Check sheet for the modelled part. Datum: model origin and axes. Units: mm. Face numbers are marked on the shaded views. A direction names the side the tool comes from. Give positions to 0.01 mm unless a question says otherwise; leave off trailing zeros. Loops run counter-clockwise (first coordinate to the right, second up) from the corner with the lowest first, then second, coordinate; pieces in that order, holes last. Notation, with made-up numbers: (55.5, 18) -> (69.5, 18) arc R37 cw to (69.5, 54) -> close; hole circle Ø6 at (23.25, 38.25). An arc over 180 degrees is marked (long way). Write each question's results on one line, items separated by ' | '. Start each with the question number.
Item 1: Cross-section at C-C on z = 18. Enter the section's corners in (x, y), then the cut area to 3 significant figures.
Item 2: Access from +Z, -Z, +X, -X, +Y, -Y to the whole of each face (thin tool, end or side, straight path). Record for the marked faces 1, 2 and 3.
Item 3: Mould release check, pull along Z, two halves, no side actions. Record for the marked faces 4, 5, 6 and 7: pulls with the +Z half, pulls with the -Z half, needs draft (parallel to the pull), parting line crosses it, or undercut.
Item 4: Cross-section at A-A on x = 57. Enter the section's corners in (y, z).
Item 5: Cross-section at D-D on x = -60. Enter the section's corners in (y, z).
Item 6: Gauge pin test, flat ends, axial feed: pin 1 Ø6 at (x, z) = (-60, 25) entering from +Y; pin 2 Ø1 at (x, z) = (51, 36) entering from +Y; pin 3 Ø1 at (y, z) = (37.5, 41.5) entering from +X; pin 4 Ø20 at (y, z) = (41.5, 14) entering from -X. Record the tip position at first contact, or that the pin passes through.
Item 7: Cross-section at B-B on z = 25. Enter the section's corners in (x, y), then the cut area to 3 significant figures.
Item 8: Scan lines: line 1 along Z through (x, y) = (-60, 1); line 2 along Y through (x, z) = (0, 24.5); line 3 along Y through (x, z) = (-20, 13). Record each from-to range of solid material in increasing order.
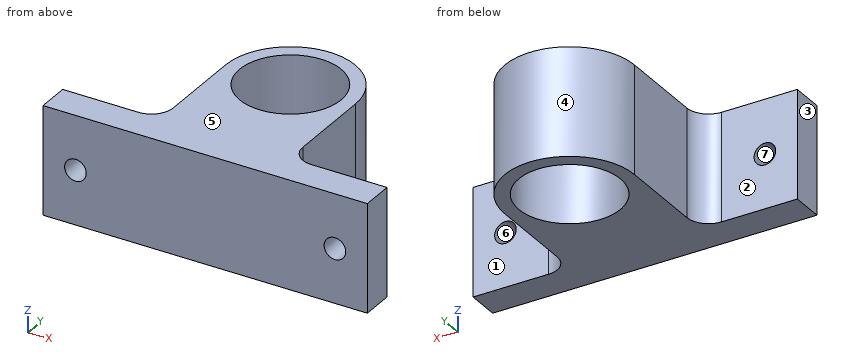
from build123d import *

# Parameters (mm, degrees)
IZIM1_R                     = 23.5
Y_KSEKLIK_EKSTR_ZYON1_DEPTH = 50
RADYUS1_R                   = 10
IZIM2_R                     = 5
KES_EKSTR_ZYON1_DEPTH       = 50


with BuildPart() as part:
    # Çizim1 → Yükseklik-Ekstrüzyon1 (new body)
    with BuildSketch(Plane.XY):
        with BuildLine():
            Line((-30, 7.5), (-30, 57.5))
            ThreePointArc((-30, 57.5), (0, 87.5), (30, 57.5))
            Line((30, 57.5), (30, 7.5))
            Line((30, 7.5), (75, 7.5))
            Line((75, 7.5), (75, -7.5))
            Line((75, -7.5), (-75, -7.5))
            Line((-75, -7.5), (-75, 7.5))
            Line((-75, 7.5), (-30, 7.5))
        make_face()
        with Locations((0, 57.5)):
            Circle(IZIM1_R, mode=Mode.SUBTRACT)
    extrude(amount=Y_KSEKLIK_EKSTR_ZYON1_DEPTH)

    # Radyus1
    radyus1_edges = [part.edges().sort_by_distance(p)[0] for p in [
        (-30, 7.5, 25),
        (30, 7.5, 25),
    ]]
    fillet(radyus1_edges, radius=RADYUS1_R)

    # Çizim2 → Kes-Ekstrüzyon1 (cut)
    with BuildSketch(Plane(origin=(0, 7.5, 0), x_dir=(1, 0, 0), z_dir=(0, 1, 0))):
        with Locations(Location((-60, -25, 0), (0, 0, 180))):
            Circle(IZIM2_R)
        with Locations(Location((60, -25, 0), (0, 0, 180))):
            Circle(IZIM2_R)
    extrude(amount=-KES_EKSTR_ZYON1_DEPTH, mode=Mode.SUBTRACT)


solid = part.part
Answer sheet:
1) outline: (-75, -7.5) -> (75, -7.5) -> (75, 7.5) -> (40, 7.5) arc R10 cw to (30, 17.5) -> (30, 57.5) arc R30 ccw to (-30, 57.5) -> (-30, 17.5) arc R10 cw to (-40, 7.5) -> (-75, 7.5) -> close; hole circle Ø47 at (0, 57.5) | area: 4,970 mm²
2) face 1: +Z, -Z, +X, +Y | face 2: +Z, -Z, -X, +Y | face 3: +Z, -Z, -X, +Y, -Y
3) face 4: needs draft | face 5: pulls with the +Z half | face 6: undercut | face 7: undercut
4) outline: (-7.5, 0) -> (7.5, 0) -> (7.5, 21) -> (-7.5, 21) -> close; (-7.5, 29) -> (7.5, 29) -> (7.5, 50) -> (-7.5, 50) -> close
5) outline: (-7.5, 0) -> (7.5, 0) -> (7.5, 20) -> (-7.5, 20) -> close; (-7.5, 30) -> (7.5, 30) -> (7.5, 50) -> (-7.5, 50) -> close
6) pin 1: passes through | pin 2: stops at y = 7.5 | pin 3: stops at x = 30 | pin 4: stops at x = -30
7) outline: (-75, -7.5) -> (-65, -7.5) -> (-65, 7.5) -> (-75, 7.5) -> close; (-55, -7.5) -> (55, -7.5) -> (55, 7.5) -> (40, 7.5) arc R10 cw to (30, 17.5) -> (30, 57.5) arc R30 ccw to (-30, 57.5) -> (-30, 17.5) arc R10 cw to (-40, 7.5) -> (-55, 7.5) -> close; (65, -7.5) -> (75, -7.5) -> (75, 7.5) -> (65, 7.5) -> close; hole circle Ø47 at (0, 57.5) | area: 4,670 mm²
8) line 1: z = 0 to 20, 30 to 50 | line 2: y = -7.5 to 34, 81 to 87.5 | line 3: y = -7.5 to 45.16, 69.84 to 79.86
